from build123d import *

# Parameters (mm, degrees)
CROQUIS3_R              = 11
CROQUIS3_R_2            = 4.5
SALIENTE_EXTRUIR2_DEPTH = 1.5
SALIENTE_EXTRUIR3_START = -1.5
CROQUIS3_3_R            = 11
SALIENTE_EXTRUIR3_DEPTH = 7
CROQUIS4_W              = 30
CROQUIS4_H              = 25
SALIENTE_EXTRUIR4_DEPTH = 8
CHAFL_N1_SIZE           = 10
CROQUIS5_R              = 2.15
CORTAR_EXTRUIR1_DEPTH   = 9
REDONDEO1_R             = 1
REDONDEO2_R             = 2
REDONDEO3_R             = 3
REDONDEO4_R             = 2
CROQUIS5_3_R            = 4
CROQUIS5_3_R_2          = 2.15
CORTAR_EXTRUIR2_DEPTH   = 1


with BuildPart() as part:
    # Croquis3 → Saliente-Extruir2 (new body)
    with BuildSketch(Plane(origin=(0, -625, 0), x_dir=(1, 0, 0), z_dir=(0, 1, 0))):
        with BuildLine():
            ThreePointArc((-40.300000436, -51), (-48.73713438, -36.15), (-40.300000436, -21.3))
            Line((-40.300000436, -21.3), (-40.300000436, 0))
            Line((-40.300000436, 0), (-10.300000436, 0))
            Line((-10.300000436, 0), (-10.300000436, -53))
            Line((-10.300000436, -53), (-40.300000436, -53))
            Line((-40.300000436, -53), (-40.300000436, -51))
        make_face()
        with Locations((-31.450000436, -36.15)):
            Circle(CROQUIS3_R, mode=Mode.SUBTRACT)
        with Locations((-31.450000436, -36.15)):
            Circle(CROQUIS3_R)
        with Locations((-31.450000436, -36.15)):
            Circle(CROQUIS3_R_2, mode=Mode.SUBTRACT)
    extrude(amount=-SALIENTE_EXTRUIR2_DEPTH)

    # Croquis3<3> → Saliente-Extruir3 (add)
    with BuildSketch(Plane(origin=(0, -625, 0), x_dir=(1, 0, 0), z_dir=(0, 1, 0)).offset(SALIENTE_EXTRUIR3_START)):
        with BuildLine():
            ThreePointArc((-40.300000436, -51), (-48.73713438, -36.15), (-40.300000436, -21.3))
            Line((-40.300000436, -21.3), (-40.300000436, 0))
            Line((-40.300000436, 0), (-10.300000436, 0))
            Line((-10.300000436, 0), (-10.300000436, -53))
            Line((-10.300000436, -53), (-40.300000436, -53))
            Line((-40.300000436, -53), (-40.300000436, -51))
        make_face()
        with Locations((-31.450000436, -36.15)):
            Circle(CROQUIS3_3_R, mode=Mode.SUBTRACT)
    extrude(amount=-SALIENTE_EXTRUIR3_DEPTH)

    # Croquis4 → Saliente-Extruir4 (add)
    with BuildSketch(Plane(origin=(0, 0, 0), x_dir=(-1, 0, 0), z_dir=(0, 0, -1))):
        with Locations((25.300000436, -646)):
            Rectangle(CROQUIS4_W, CROQUIS4_H)
    extrude(amount=-SALIENTE_EXTRUIR4_DEPTH)

    # Chaflán1
    chafl_n1_edges = [part.edges().sort_by_distance(p)[0] for p in [
        (-25.300000436, -633.5, 8),
    ]]
    chamfer(chafl_n1_edges, length=CHAFL_N1_SIZE)

    # Croquis5 → Cortar-Extruir1 (cut, through all)
    with BuildSketch(Plane.XY.offset(8)):
        with Locations((-25.300000436, -651)):
            Circle(CROQUIS5_R)
    extrude(amount=-CORTAR_EXTRUIR1_DEPTH, mode=Mode.SUBTRACT)

    # Redondeo1
    redondeo1_edges = [part.edges().sort_by_distance(p)[0] for p in [
        (-40.300000436, -629.25, 53),
        (-40.300000436, -629.25, 51),
    ]]
    fillet(redondeo1_edges, radius=REDONDEO1_R)

    # Redondeo2
    redondeo2_edges = [part.edges().sort_by_distance(p)[0] for p in [
        (-10.300000436, -629.25, 53),
    ]]
    fillet(redondeo2_edges, radius=REDONDEO2_R)

    # Redondeo3
    redondeo3_edges = [part.edges().sort_by_distance(p)[0] for p in [
        (-25.300000436, -633.5, 18),
        (-25.300000436, -643.5, 8),
    ]]
    fillet(redondeo3_edges, radius=REDONDEO3_R)

    # Redondeo4
    redondeo4_edges = [part.edges().sort_by_distance(p)[0] for p in [
        (-25.300000436, -658.5, 8),
    ]]
    fillet(redondeo4_edges, radius=REDONDEO4_R)

    # Croquis5<3> → Cortar-Extruir2 (cut)
    with BuildSketch(Plane.XY.offset(8)):
        with Locations((-25.300000436, -651)):
            Circle(CROQUIS5_3_R)
        with Locations((-25.300000436, -651)):
            Circle(CROQUIS5_3_R_2, mode=Mode.SUBTRACT)
    extrude(amount=-CORTAR_EXTRUIR2_DEPTH, mode=Mode.SUBTRACT)


solid = part.part
Read the model definition and answer for the solid it produces. Units are mm, in the model's axes. A direction names the side the tool comes from. Coordinates: 2 decimals unless noted, no trailing zeros. Loops run counter-clockwise (first coordinate to the right, second up) from the corner with the lowest first, then second, coordinate; pieces in that order, holes last.
Q1. Which of the six approach directions +Z, -Z, +X, -X, +Y, -Y give full straight-line access (tool end or side, diameter ignored) to faces 1 (the face through (-10.3, -633, 16)), 2 (the face through (-26.167, -654.905, 7.507)), 3 (the face through (-25.1, -646.6, 8)), 4 (the face through (-25, -658.5, 3)), 5 (the face through (-40.3, -638, 8))?
Q2. The part is cut by section D-D on y = -630. Write down the section's boundary in (x, z).
Q3. The mould has two halves that part along Z. Classify faces 6 (the face through (-48.737, -629.19, 36.125)), 7 (the face through (-26.374, -629.951, 45.909)), 8 (the face through (-25, -642, 0)), 9 (the face through (-24, -653, 7)): +Z half, -Z half, draft (parallel to the pull), parting line (faces both ways), or undercut.
Q4. The part is cut by section B-B on x = -31.45. Write down the section's boundary in (y, z).
Q5. Each of these flat-tipped pins is pushed along its axis until it touches: pin 1 Ø9.5 at (x, y) = (-21, -648) entering from +Z; pin 2 Ø11 at (x, z) = (-35, 41) entering from -Y; pin 3 Ø2.5 at (x, y) = (-25.3, -651) entering from +Z; pin 4 Ø0.5 at (y, z) = (-630, 51.5) entering from -X. Where does it stop, or does it pass through?
Q6. The part is cut by section A-A on z = 36.15. Write down the section's boundary in (x, y), and give its area (3 significant figures).
Q7. The part is cut by section C-C on y = -651. Write down the section's boundary in (x, z), and give its area (3 significant figures).
Q8. Consider probe 1 along X at (y, z) = (-651, 7.7); probe 2 along Z at (x, y) = (-31.45, -625.45); probe 3 along X at (y, z) = (-628.75, 36.15). Determine where each line is inside the solid, lowest interval first.
Results below:
1. face 1: +Z, -Z, +X, +Y, -Y
1. face 2: +Z
1. face 3: +Z, +X, -X, -Y
1. face 4: +Z, -Z, +X, -X, -Y
1. face 5: -Z, -X, +Y, -Y
2. outline: (-40.76, 50.72) arc R17.29 ccw to (-40.3, 21.3) - (-40.3, 0) - (-10.3, 0) - (-10.3, 51) arc R2 ccw to (-12.3, 53) - (-39.3, 53) arc R1 ccw to (-40.3, 52) - (-40.3, 51.56) arc R1 cw to start; hole circle Ø22 at (-31.45, 36.15)
3. face 6: parting line
3. face 7: undercut
3. face 8: -Z half
3. face 9: +Z half
4. outline: (-658.5, 0) - (-625, 0) - (-625, 31.65) - (-626.5, 31.65) - (-626.5, 25.15) - (-633.5, 25.15) - (-633.5, 19.24) arc R3 cw to (-634.38, 17.12) - (-642.62, 8.88) arc R3 cw to (-644.74, 8) - (-656.5, 8) arc R2 ccw to (-658.5, 6) - close; (-633.5, 47.15) - (-626.5, 47.15) - (-626.5, 40.65) - (-625, 40.65) - (-625, 53) - (-633.5, 53) - close
5. pin 1: stops at z = 8.4
5. pin 2: stops at y = -633.5
5. pin 3: passes through
5. pin 4: stops at x = -40.35
6. outline: (-48.74, -633.5) - (-42.45, -633.5) - (-42.45, -626.5) - (-35.95, -626.5) - (-35.95, -625) - (-48.74, -625) - close; (-26.95, -626.5) - (-20.45, -626.5) - (-20.45, -633.5) - (-10.3, -633.5) - (-10.3, -625) - (-26.95, -625) - close
6. area: 159 mm2
7. outline: (-40.3, 0) - (-27.45, 0) - (-27.45, 7) - (-29.3, 7) - (-29.3, 8) - (-40.3, 8) - close; (-23.15, 0) - (-10.3, 0) - (-10.3, 8) - (-21.3, 8) - (-21.3, 7) - (-23.15, 7) - close
7. area: 202 mm2
8. probe 1: x = -40.3 to -29.3, -21.3 to -10.3
8. probe 2: z = 0 to 31.65, 40.65 to 53
8. probe 3: x = -48.74 to -42.45, -20.45 to -10.3
